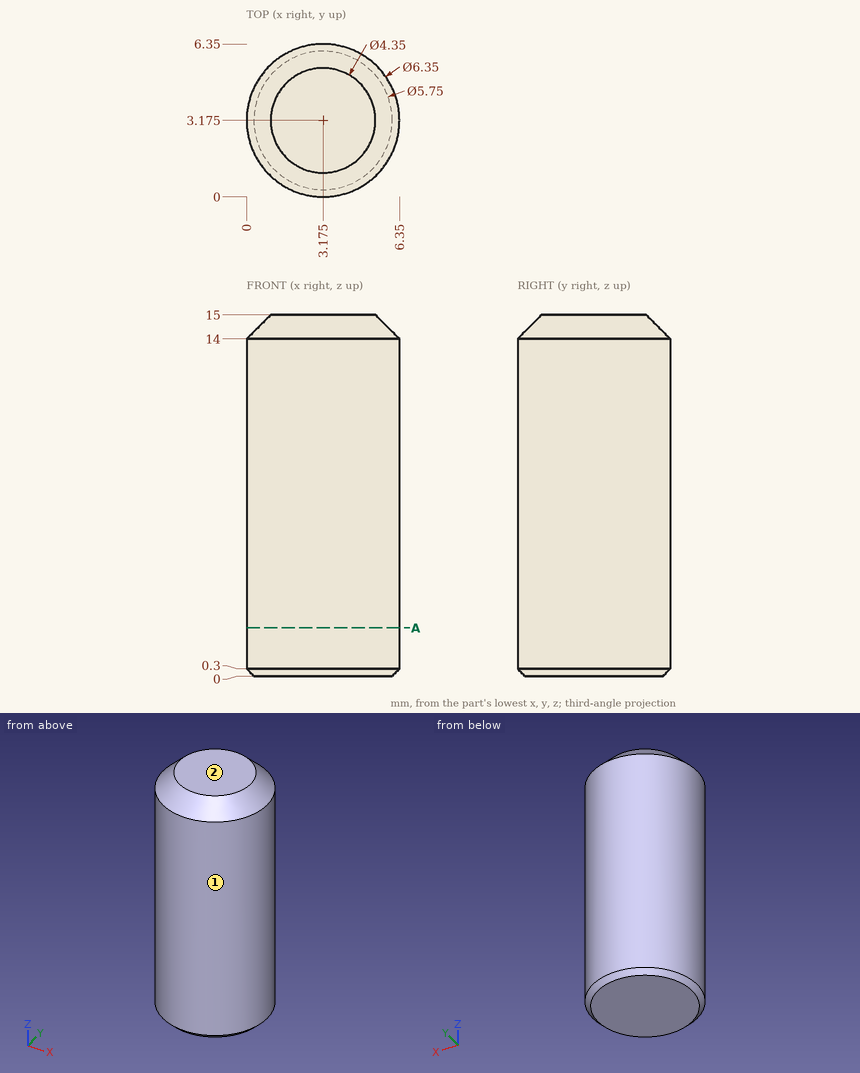
Source: three-view drawing plus pictorial views. Frame: mm from the lowest corner of the part. Round coordinates to 2 decimals unless told otherwise and drop trailing zeros. Write each loop counter-clockwise with the first axis right and the second up, starting at its lowest first coordinate (ties: lowest second). Pieces come first, ordered by that corner, then holes. Notation, with made-up numbers: M 60.25,81.5 L 105.25,81.5 A12 cw 105.25,86.5 Z; hole C -22,72.25 d10. An arc over 180 degrees is marked long. Use CSV: the item, a comma, the result in double quotes. Start each with the question number.
Q1. Line query: line 1 (Y direction, x = 2, z = 2.5); line 2 (Y direction, x = 3.25, z = 12.5); line 3 (Z direction, x = 4.25, y = 1.25). Output: solid intervals per line, ascending. Write a range as from..to.
Q2. Cut plane A-A on z = 2. Output: boundary loops of the cut face in (x, y) (3 decimals), plus the area to 3 significant figures.
Q3. First-contact query: P1, Ø1, axis at y = 1.5, z = 2.5, coming from the -X side; P2, Ø1, axis at x = 4.5, z = 11, coming from the -Y side; P3, Ø2, axis at x = 1.5, z = 13, coming from the +Y side. Flat tips, straight axial feed; report the tip coordinate or a pass-through.
Q4. Pull-direction query (X, two-part tool) for the marked faces 1 and 2; classes: +X half, -X half, draft (parallel to the pull), parting line (faces both ways), or undercut.
Results found:
1,line 1,"0.23..6.12"
1,line 2,"0..6.35"
1,line 3,"0..14.97"
2,outline,"C 3.175,3.175 d6.35"
2,area,"31.7 mm^2"
3,P1,"x = 0.23"
3,P2,"y = 0.11"
3,P3,"y = 6.28"
4,face 1,"parting line"
4,face 2,"draft"
